Drawing for the job (mm, zero at the part's lowest x, y, z). A direction names the side the tool comes from. Round coordinates to 2 decimals unless told otherwise and drop trailing zeros. Write each loop counter-clockwise with the first axis right and the second up, starting at its lowest first coordinate (ties: lowest second). Pieces come first, ordered by that corner, then holes.
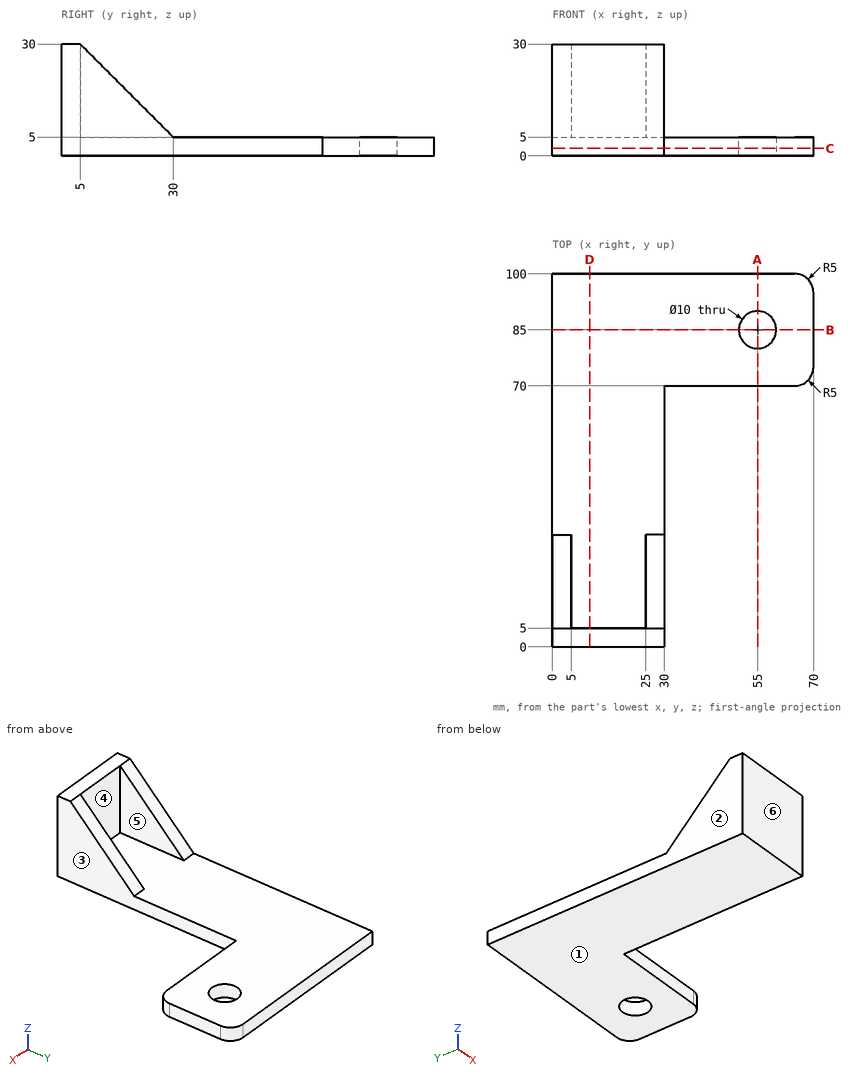
1) Cut at A-A on x = 55. List the corners of the cut face in (y, z).
2) Flat gauge pins, fed straight in: pin 1 Ø6 at (x, y) = (59, 66) entering from -Z; pin 2 Ø16 at (x, z) = (14, 17) entering from +Y; pin 3 Ø15 at (y, z) = (22, 14.5) entering from +X; pin 4 Ø5.5 at (x, z) = (54, 1.5) entering from -Y. Where does each tip first touch, or does it go through?
3) Which spindle directions (+Z, -Z, +X, -X, +Y, -Y) get a long thin tool onto all of the face, cutting with end or side? Do the marked faces 5 and 6. Say none if no direction does.
4) Cut at B-B on y = 85. List the corners of the cut face in (x, z).
5) Cut at D-D on x = 10. List the corners of the cut face in (y, z).
6) Cut at C-C on z = 2. List the corners of the cut face in (x, y).
7) Pull direction X, two halves, no side cores. Call the marked faces 1, 2, 3 and 4: released by +X, released by -X, zero draft, split by the parting line, or undercut.
8) Wall check: probe 1 along Y at (x, z) = (55, 2); probe 2 along Z at (x, y) = (8, 82). Give the ranges that are in metal, low to high.
Result sheet:
1. outline: (70, 0) - (80, 0) - (80, 5) - (70, 5) - close; (90, 0) - (100, 0) - (100, 5) - (90, 5) - close
2. pin 1: passes through
2. pin 2: stops at y = 5
2. pin 3: stops at x = 30
2. pin 4: stops at y = 70
3. face 5: +Z, +Y
3. face 6: +Z, -Z, +X, -X, -Y
4. outline: (0, 0) - (50, 0) - (50, 5) - (0, 5) - close; (60, 0) - (70, 0) - (70, 5) - (60, 5) - close
5. outline: (0, 0) - (100, 0) - (100, 5) - (5, 5) - (5, 30) - (0, 30) - close
6. outline: (0, 0) - (30, 0) - (30, 70) - (65, 70) arc R5 ccw to (70, 75) - (70, 95) arc R5 ccw to (65, 100) - (0, 100) - close; hole circle Ø10 at (55, 85)
7. face 1: zero draft
7. face 2: released by -X
7. face 3: released by +X
7. face 4: undercut
8. probe 1: y = 70 to 80, 90 to 100
8. probe 2: z = 0 to 5
